Geometry: final body of the model. Coordinates: model frame, mm. A direction names the side the tool comes from. Give positions to 0.01 mm unless a question says otherwise; leave off trailing zeros. Write each loop counter-clockwise with the first axis right and the second up, starting at its lowest first coordinate (ties: lowest second). Pieces come first, ordered by that corner, then holes.
from build123d import *

# Parameters (mm, degrees)
F1_DEPTH  = 8
F2_R      = 2.25
F3_DEPTH  = 2
F5_DEPTH  = 2
F7_DEPTH  = 2
F2_R_2    = 4
F8_DEPTH  = 4.4
F9_DEPTH  = 8.001
F10_DEPTH = 8.001
F11_DEPTH = 4.4


# Not quite as in the source:
# - a feature names something its author has since deleted; it is built from what else it names


with BuildPart() as f1:
    # F0 (on Front) → F1 (new body)
    with BuildSketch(Plane.XZ):
        Polygon((24, 31.5), (0, 31.5), (-24, 31.5), (-24, -31.5), (0, -31.5), (24, -31.5), align=None)
    extrude(amount=F1_DEPTH)

    # F2 (on face) → F3 (cut)
    with BuildSketch(Plane.XZ.offset(8)):
        with Locations((-19, 26.5)):
            Circle(F2_R)
        with Locations((19, 26.5)):
            Circle(F2_R)
    extrude(amount=-F3_DEPTH, mode=Mode.SUBTRACT)

    # F4 (on face) → F5 (cut)
    with BuildSketch(Plane.XZ.offset(8)):
        with BuildLine():
            Line((-11, -28.5), (0, -28.5))
            Line((0, -28.5), (11, -28.5))
            ThreePointArc((11, -28.5), (12.4142135624, -27.9142135624), (13, -26.5))
            ThreePointArc((13, -26.5), (14.7573593129, -22.2573593129), (19, -20.5))
            ThreePointArc((19, -20.5), (20.4142135624, -19.9142135624), (21, -18.5))
            Line((21, -18.5), (21, 0))
            Line((21, 0), (21, 18.5))
            ThreePointArc((21, 18.5), (20.4142135624, 19.9142135624), (19, 20.5))
            ThreePointArc((19, 20.5), (14.7573593129, 22.2573593129), (13, 26.5))
            ThreePointArc((13, 26.5), (12.4142135624, 27.9142135624), (11, 28.5))
            Line((11, 28.5), (0, 28.5))
            Line((0, 28.5), (-11, 28.5))
            ThreePointArc((-11, 28.5), (-12.4142135624, 27.9142135624), (-13, 26.5))
            ThreePointArc((-13, 26.5), (-14.7573593129, 22.2573593129), (-19, 20.5))
            ThreePointArc((-19, 20.5), (-20.4142135624, 19.9142135624), (-21, 18.5))
            Line((-21, 18.5), (-21, 0))
            Line((-21, 0), (-21, -18.5))
            ThreePointArc((-21, -18.5), (-20.4142135624, -19.9142135624), (-19, -20.5))
            ThreePointArc((-19, -20.5), (-14.7573593129, -22.2573593129), (-13, -26.5))
            ThreePointArc((-13, -26.5), (-12.4142135624, -27.9142135624), (-11, -28.5))
        make_face()
    extrude(amount=-F5_DEPTH, mode=Mode.SUBTRACT)

    # F6 (on face) → F7 (join)
    with BuildSketch(Plane.XZ.offset(6)):
        Polygon((-9.214199551, -4.3776710518), (-8.2052831758, -4.3776710518), (-8.2052831758, 4.3035698491), (-9.214199551, 4.3035698491), (-9.214199551, 0.6099098991), (-13.7875737792, 0.6099098991), (-13.7875737792, 4.3035698491), (-14.7964901544, 4.3035698491), (-14.7964901544, -4.3776710518), (-13.7875737792, -4.3776710518), (-13.7875737792, -0.2926047491), (-9.214199551, -0.2926047491), align=None)
        with BuildLine():
            Line((-3.9055133884, -4.3776710518), (-2.9079971982, -4.3776710518))
            Line((-2.9079971982, -4.3776710518), (0.2194535618, 4.3035698491))
            Line((0.2194535618, 4.3035698491), (-0.8654640469, 4.3035698491))
            Line((-0.8654640469, 4.3035698491), (-2.8490962422, -1.2787207543))
            add(Edge.make_bspline(
                [(-3.4077053087, -3.1958518703), (-3.193001824, -2.234436266), (-2.8490962422, -1.2787207543)],
                knots=[0, 0, 0, 1, 1, 1], degree=2))
            add(Edge.make_bspline(
                [(-3.9530141594, -1.3129213094), (-3.6091085776, -2.281937037), (-3.4077053087, -3.1958518703)],
                knots=[0, 0, 0, 1, 1, 1], degree=2))
            Line((-3.9530141594, -1.3129213094), (-5.9480465397, 4.3035698491))
            Line((-5.9480465397, 4.3035698491), (-7.0177639018, 4.3035698491))
            Line((-7.0177639018, 4.3035698491), (-3.9055133884, -4.3776710518))
        make_face()
        with BuildLine():
            add(Edge.make_bspline(
                [(3.8245554648, -4.3776710518), (2.7125988005, -4.1239843021), (2.0045325346, -3.3326540906)],
                knots=[0.3205826669, 0.3205826669, 0.3205826669, 1, 1, 1], degree=2))
            Line((3.8245554648, -4.3776710518), (6.3867026136, -4.3776710518))
            add(Edge.make_bspline(
                [(7.1906667081, -4.1572674745), (6.8235762872, -4.2956026015), (6.3867026136, -4.3776710518)],
                knots=[0, 0, 0, 0.406741787, 0.406741787, 0.406741787], degree=2))
            Line((7.1906667081, -4.1572674745), (7.1906667081, -3.2737531346))
            add(Edge.make_bspline(
                [(5.1177330633, -3.6005584388), (6.0259478041, -3.6005584388), (7.1906667081, -3.2737531346)],
                knots=[0, 0, 0, 1, 1, 1], degree=2))
            add(Edge.make_bspline(
                [(2.8405461035, -2.6704933434), (3.639509071, -3.6005584388), (5.1177330633, -3.6005584388)],
                knots=[0, 0, 0, 1, 1, 1], degree=2))
            add(Edge.make_bspline(
                [(2.0415831359, -0.0380006168), (2.0415831359, -1.740428248), (2.8405461035, -2.6704933434)],
                knots=[0, 0, 0, 1, 1, 1], degree=2))
            add(Edge.make_bspline(
                [(2.8699965815, 2.5716917398), (2.0415831359, 1.6188262744), (2.0415831359, -0.0380006168)],
                knots=[0, 0, 0, 1, 1, 1], degree=2))
            add(Edge.make_bspline(
                [(5.1291332484, 3.5245572053), (3.698410027, 3.5245572053), (2.8699965815, 2.5716917398)],
                knots=[0, 0, 0, 1, 1, 1], degree=2))
            add(Edge.make_bspline(
                [(7.1013652587, 3.0628497116), (6.1152492535, 3.5245572053), (5.1291332484, 3.5245572053)],
                knots=[0, 0, 0, 1, 1, 1], degree=2))
            Line((7.1013652587, 3.0628497116), (7.5288721973, 3.9292637739))
            add(Edge.make_bspline(
                [(5.9680043466, 4.3776710518), (6.8286727205, 4.2702531102), (7.5288721973, 3.9292637739)],
                knots=[0.3150184776, 0.3150184776, 0.3150184776, 1, 1, 1], degree=2))
            Line((5.9680043466, 4.3776710518), (4.4013922849, 4.3776710518))
            add(Edge.make_bspline(
                [(2.9127472753, 3.8808129875), (3.5750775116, 4.2627988309), (4.4013922849, 4.3776710518)],
                knots=[0, 0, 0, 0.6992762354, 0.6992762354, 0.6992762354], degree=2))
            add(Edge.make_bspline(
                [(1.463973761, 2.3256377463), (1.9655819024, 3.3345541215), (2.9127472753, 3.8808129875)],
                knots=[0, 0, 0, 1, 1, 1], degree=2))
            add(Edge.make_bspline(
                [(0.9623656197, -0.0247004009), (0.9623656197, 1.316721371), (1.463973761, 2.3256377463)],
                knots=[0, 0, 0, 1, 1, 1], degree=2))
            add(Edge.make_bspline(
                [(2.0045325346, -3.3326540906), (0.9623656197, -2.1679351867), (0.9623656197, -0.0247004009)],
                knots=[0, 0, 0, 1, 1, 1], degree=2))
        make_face()
        with BuildLine():
            add(Edge.make_bspline(
                [(11.4968799904, -4.3776710518), (10.3849233261, -4.1239843021), (9.6768570602, -3.3326540906)],
                knots=[0.3205826669, 0.3205826669, 0.3205826669, 1, 1, 1], degree=2))
            Line((11.4968799904, -4.3776710518), (14.0590271393, -4.3776710518))
            add(Edge.make_bspline(
                [(14.8629912337, -4.1572674745), (14.4959008129, -4.2956026015), (14.0590271393, -4.3776710518)],
                knots=[0, 0, 0, 0.406741787, 0.406741787, 0.406741787], degree=2))
            Line((14.8629912337, -4.1572674745), (14.8629912337, -3.2737531346))
            add(Edge.make_bspline(
                [(12.790057589, -3.6005584388), (13.6982723297, -3.6005584388), (14.8629912337, -3.2737531346)],
                knots=[0, 0, 0, 1, 1, 1], degree=2))
            add(Edge.make_bspline(
                [(10.5128706291, -2.6704933434), (11.3118335967, -3.6005584388), (12.790057589, -3.6005584388)],
                knots=[0, 0, 0, 1, 1, 1], degree=2))
            add(Edge.make_bspline(
                [(9.7139076615, -0.0380006168), (9.7139076615, -1.740428248), (10.5128706291, -2.6704933434)],
                knots=[0, 0, 0, 1, 1, 1], degree=2))
            add(Edge.make_bspline(
                [(10.5423211071, 2.5716917398), (9.7139076615, 1.6188262744), (9.7139076615, -0.0380006168)],
                knots=[0, 0, 0, 1, 1, 1], degree=2))
            add(Edge.make_bspline(
                [(12.801457774, 3.5245572053), (11.3707345527, 3.5245572053), (10.5423211071, 2.5716917398)],
                knots=[0, 0, 0, 1, 1, 1], degree=2))
            add(Edge.make_bspline(
                [(14.7736897843, 3.0628497116), (13.7875737792, 3.5245572053), (12.801457774, 3.5245572053)],
                knots=[0, 0, 0, 1, 1, 1], degree=2))
            Line((14.7736897843, 3.0628497116), (15.201196723, 3.9292637739))
            add(Edge.make_bspline(
                [(13.6403288722, 4.3776710518), (14.5009972462, 4.2702531102), (15.201196723, 3.9292637739)],
                knots=[0.3150184776, 0.3150184776, 0.3150184776, 1, 1, 1], degree=2))
            Line((13.6403288722, 4.3776710518), (12.0737168105, 4.3776710518))
            add(Edge.make_bspline(
                [(10.585071801, 3.8808129875), (11.2474020372, 4.2627988309), (12.0737168105, 4.3776710518)],
                knots=[0, 0, 0, 0.6992762354, 0.6992762354, 0.6992762354], degree=2))
            add(Edge.make_bspline(
                [(9.1362982866, 2.3256377463), (9.637906428, 3.3345541215), (10.585071801, 3.8808129875)],
                knots=[0, 0, 0, 1, 1, 1], degree=2))
            add(Edge.make_bspline(
                [(8.6346901453, -0.0247004009), (8.6346901453, 1.316721371), (9.1362982866, 2.3256377463)],
                knots=[0, 0, 0, 1, 1, 1], degree=2))
            add(Edge.make_bspline(
                [(9.6768570602, -3.3326540906), (8.6346901453, -2.1679351867), (8.6346901453, -0.0247004009)],
                knots=[0, 0, 0, 1, 1, 1], degree=2))
        make_face()
        with BuildLine():
            Line((6.3867026136, -4.3776710518), (3.8245554648, -4.3776710518))
            add(Edge.make_bspline(
                [(4.9638305654, -4.4973729946), (4.3492315594, -4.4973729946), (3.8245554648, -4.3776710518)],
                knots=[0, 0, 0, 0.3205826669, 0.3205826669, 0.3205826669], degree=2))
            add(Edge.make_bspline(
                [(6.3867026136, -4.3776710518), (5.7494951686, -4.4973729946), (4.9638305654, -4.4973729946)],
                knots=[0.406741787, 0.406741787, 0.406741787, 1, 1, 1], degree=2))
        make_face()
        with BuildLine():
            Line((14.0590271393, -4.3776710518), (11.4968799904, -4.3776710518))
            add(Edge.make_bspline(
                [(12.6361550911, -4.4973729946), (12.0215560851, -4.4973729946), (11.4968799904, -4.3776710518)],
                knots=[0, 0, 0, 0.3205826669, 0.3205826669, 0.3205826669], degree=2))
            add(Edge.make_bspline(
                [(14.0590271393, -4.3776710518), (13.4218196942, -4.4973729946), (12.6361550911, -4.4973729946)],
                knots=[0.406741787, 0.406741787, 0.406741787, 1, 1, 1], degree=2))
        make_face()
        with BuildLine():
            add(Edge.make_bspline(
                [(4.4013922849, 4.3776710518), (4.7567489763, 4.4270718536), (5.1424334642, 4.4270718536)],
                knots=[0.6992762354, 0.6992762354, 0.6992762354, 1, 1, 1], degree=2))
            Line((4.4013922849, 4.3776710518), (5.9680043466, 4.3776710518))
            add(Edge.make_bspline(
                [(5.1424334642, 4.4270718536), (5.5721886465, 4.4270718536), (5.9680043466, 4.3776710518)],
                knots=[0, 0, 0, 0.3150184776, 0.3150184776, 0.3150184776], degree=2))
        make_face()
        with BuildLine():
            Line((12.0737168105, 4.3776710518), (13.6403288722, 4.3776710518))
            add(Edge.make_bspline(
                [(12.8147579899, 4.4270718536), (13.2445131721, 4.4270718536), (13.6403288722, 4.3776710518)],
                knots=[0, 0, 0, 0.3150184776, 0.3150184776, 0.3150184776], degree=2))
            add(Edge.make_bspline(
                [(12.0737168105, 4.3776710518), (12.4290735019, 4.4270718536), (12.8147579899, 4.4270718536)],
                knots=[0.6992762354, 0.6992762354, 0.6992762354, 1, 1, 1], degree=2))
        make_face()
    extrude(amount=F7_DEPTH)

    # F2 (on face) → F8 (cut)
    with BuildSketch(Plane.XZ.offset(8)):
        with Locations((-19, 26.5)):
            Circle(F2_R_2)
        with Locations((-19, 26.5)):
            Circle(F2_R, mode=Mode.SUBTRACT)
        with Locations((19, 26.5)):
            Circle(F2_R_2)
        with Locations((19, 26.5)):
            Circle(F2_R, mode=Mode.SUBTRACT)
    extrude(amount=-F8_DEPTH, mode=Mode.SUBTRACT)

    # F2 (on face) → F9 (cut, through all)
    with BuildSketch(Plane.XZ.offset(8)):
        with Locations((-19, 26.5)):
            Circle(F2_R)
        with Locations((19, 26.5)):
            Circle(F2_R)
    extrude(amount=-F9_DEPTH, mode=Mode.SUBTRACT)

    # F2 (on face) → F10 (cut, through all)
    with BuildSketch(Plane.XZ.offset(8)):
        with Locations((-19, -26.5)):
            Circle(F2_R)
        with Locations((19, -26.5)):
            Circle(F2_R)
    extrude(amount=-F10_DEPTH, mode=Mode.SUBTRACT)

    # F2 (on face) → F11 (cut)
    with BuildSketch(Plane.XZ.offset(8)):
        with Locations((-19, -26.5)):
            Circle(F2_R_2)
        with Locations((-19, -26.5)):
            Circle(F2_R, mode=Mode.SUBTRACT)
        with Locations((19, -26.5)):
            Circle(F2_R_2)
        with Locations((19, -26.5)):
            Circle(F2_R, mode=Mode.SUBTRACT)
    extrude(amount=-F11_DEPTH, mode=Mode.SUBTRACT)


solid = f1.part
Q1. Section A-A on y = -4.25. Output: boundary loops of the cut face in (x, z).
Filled sheet:
outline: (-24, -31.5) - (24, -31.5) - (24, 31.5) - (-24, 31.5) - close; hole circle Ø8 at (-19, -26.5); hole circle Ø8 at (-19, 26.5); hole circle Ø8 at (19, -26.5); hole circle Ø8 at (19, 26.5)
Q2. Pull-direction query (Z, two-part tool) for faces 1 (the flat face through (-12, -8, 0)), 2 (the flat face through (-14.796, -7, 0)); classes: released by +Z, released by -Z, zero draft, split by the parting line, or undercut.
Filled sheet:
face 1: zero draft
face 2: undercut
Q3. Section C-C on z = 25.5. Output: boundary loops of the cut face in (x, y), plus the area to 3 significant figures.
Filled sheet:
outline: (-24, -8) - (-22.87, -8) - (-22.87, -3.6) - (-21.02, -3.6) - (-21.02, 0) - (-24, 0) - close; (-16.98, -3.6) - (-15.13, -3.6) - (-15.13, -8) - (-13.08, -8) - (-13.08, -6) - (13.08, -6) - (13.08, -8) - (15.13, -8) - (15.13, -3.6) - (16.98, -3.6) - (16.98, 0) - (-16.98, 0) - close; (21.02, -3.6) - (22.87, -3.6) - (22.87, -8) - (24, -8) - (24, 0) - (21.02, 0) - close
area: 234 mm2
Q4. Ray query, line 1 along Z through (x, y) = (-19, -5.85); line 2 along Z through (x, y) = (19, -2.35); line 3 along X through (y, z) = (-7.5, -27.5). Return the intervals inside material, ascending.
Filled sheet:
line 1: z = -31.5 to -30.5, -22.5 to 22.5, 30.5 to 31.5
line 2: z = -31.5 to -28.75, -24.25 to 24.25, 28.75 to 31.5
line 3: x = -24 to -22.87, -15.13 to -12.73, 12.73 to 15.13, 22.87 to 24
Q5. Access query for faces 3 (the flat face through (-9.214, -7, -2)), 4 (the cylindrical face through (-17.962, -1.825, 24.504)). Directions: +Z, -Z, +X, -X, +Y, -Y. A direction counts if a zero-diameter tool reaches every point of the face in a straight line with its end or side. Return the directions, or none.
Filled sheet:
face 3: -Y
face 4: +Y, -Y
Q6. Pin query (flat end, axial travel): P1, Ø2.5, axis at x = 21, z = -27.5, coming from the -Y side; P2, Ø4, axis at x = 10.5, z = 15.5, coming from the -Y side. Return the tip coordinate at first contact, or that it passes through.
Filled sheet:
P1: stops at y = -3.6
P2: stops at y = -6
Q7. Section B-B on z = -13.5. Output: boundary loops of the cut face in (x, y), plus the area to 3 significant figures.
Filled sheet:
outline: (-24, -8) - (-21, -8) - (-21, -6) - (21, -6) - (21, -8) - (24, -8) - (24, 0) - (-24, 0) - close
area: 300 mm2
